Build history of the part. All positions in model axes, mm. Coordinates: 2 decimals unless noted, no trailing zeros. Write each loop counter-clockwise with the first axis right and the second up, starting at its lowest first coordinate (ties: lowest second). Pieces come first, ordered by that corner, then holes.
Autodesk Inventor part; units mm, degrees
ref_plane "YZ Plane" through (0, 0, 0) normal (1, 0, 0) x (0, 1, 0)
ref_plane "XZ Plane" through (0, 0, 0) normal (0, 1, 0) x (-1, 0, 0)
ref_plane "XY Plane" through (0, 0, 0) normal (0, 0, 1) x (1, 0, 0)
sketch "Sketch3" plane through (0, 0, 0) normal (0, 1, 0) x (-1, 0, 0)
  line L0 (0, 0) -> (-1104, 0)
  line L1 (-1104, 0) -> (-1104, -50)
  line L2 (-1104, -50) -> (0, -50)
  line L3 (0, -50) -> (0, 0)
  dimension "d25" = 50
  dimension "d28" = 1104
extrude "Plate3" add sketch "Sketch3" along normal blind 2
sketch "Sketch4" plane through (1104, 2, -48) normal (0, 0, -1) x (-1, 0, 0)
  line L0 (1104, 0) -> (0, 0)
  line L1 (0, 0) -> (0, -20)
  line L2 (0, -20) -> (1104, -20)
  line L3 (1104, -20) -> (1104, 0)
edge flange "Flange2" height 20 angle 90 thickness 2 bend radius 2 thickness toward (0, 0, -1) relief tear relief width 2 relief depth 1 edges at (552, 0, -50) wall of the first edge with corners at (0, 2, -48) (1104, 2, -48) (1104, -18, -48) (0, -18, -48)
bend "Bend3"
corner "Corner3"
equation "\"d30\" = Thickness"
equation "\"d31\" = BendReliefWidth"
equation "\"d32\" = BendReliefDepth"
equation "\"d33\" = MinimumRemnant"
equation "\"d34\" = TransitionRadius"
equation "\"d37\" = BendRadius"
equation "\"d38\" = CornerReliefSize"
equation "\"d39\" = GapSize"
equation "\"d40\" = JacobiRadiusSize"
equation "\"BendRadius\" = Thickness"
equation "\"BendReliefWidth\" = Thickness"
equation "\"BendReliefDepth\" = 0.5 * Thickness"
equation "\"CornerReliefSize\" = 4 * Thickness"
equation "\"MinimumRemnant\" = 2 * Thickness"
equation "\"TransitionRadius\" = BendRadius"
equation "\"JacobiRadiusSize\" = BendRadius"
equation "\"GapSize\" = Thickness"
properties part number "GBK-RK-0043 rib 3"
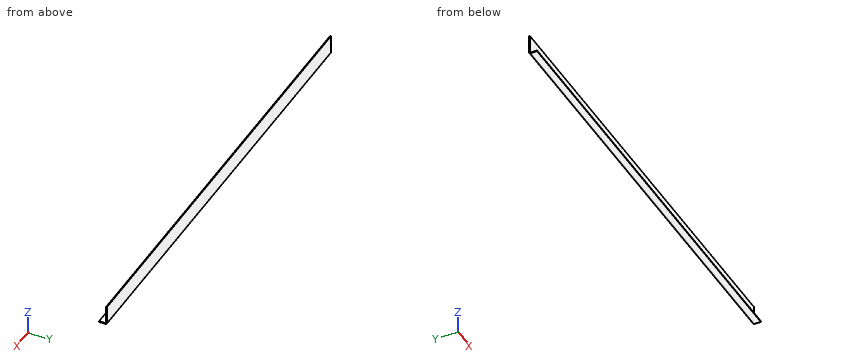
1. Saw through at A-A on x = 219.5. List the corners of the cut face in (y, z), plus the area to 3 significant figures.
Computed values:
outline: (-18, -50) - (-2, -50) arc R4 ccw to (2, -46) - (2, 0) - (0, 0) - (0, -46) arc R2 cw to (-2, -48) - (-18, -48) - close
area: 133 mm2
2. Saw through at C-C on z = -37. List the corners of the cut face in (x, y), plus the area to 3 significant figures.
Computed values:
outline: (0, 0) - (1104, 0) - (1104, 2) - (0, 2) - close
area: 2,210 mm2
3. Saw through at B-B on y = -9. List the corners of the cut face in (x, z), plus the area to 3 significant figures.
Computed values:
outline: (0, -50) - (1104, -50) - (1104, -48) - (0, -48) - close
area: 2,210 mm2
4. Flat gauge pins, fed straight in: pin 1 (23 mm diameter, centred on x = 585.5, z = -32, fed in from -Y); pin 2 (8 mm diameter, centred on x = 319.5, y = -12.5, fed in from +Z). Where does each tip first touch, or does it go through?
Computed values:
pin 1: stops at y = 0
pin 2: stops at z = -48
5. Probe line 1 along Z through (x, y) = (436.5, -17); line 2 along Y through (x, z) = (782, -27.5); line 3 along Z through (x, y) = (283, -0.5). List the from-to ranges inside material, lowest first.
Computed values:
line 1: z = -50 to -48
line 2: y = 0 to 2
line 3: z = -49.71 to -47.32
